Source: CAD feature listing. Evaluate the final solid. Frame: model axes, mm. A direction names the side the tool comes from. Give positions to 0.01 mm unless a question says otherwise; leave off trailing zeros. Order: outer loops, then holes, each group sorted by start corner. A loop starts at its lowest first (then second) coordinate and runs counter-clockwise, first axis right, second up. Notation, with made-up numbers: M 63.5,1 L 102.5,1 A28 cw 102.5,33 Z; hole C -8,-13 d3. An arc over 180 degrees is marked long. Answer as a JSON object with one key per item and string values. Group by question number.
1. Set-up query: faces 1 (the cylindrical face through (-2.17, -27.32, -54.76)), 2 (the flat face through (0, 0, 5)), 3 (the flat face through (4, 7, 205)). Return all of +Z, -Z, +X, -X, +Y, -Y with unobstructed straight access to the full face (end or side cutting, diameter ignored); none if empty.
2. Section query D-D (y = -28.5). Output: boundary loops of the cut face in (x, z), plus the area to 3 significant figures.
3. Section query B-B (y = 0). Output: boundary loops of the cut face in (x, z), plus the area to 3 significant figures.
4. Pin query (flat end, axial travel): P1, Ø1, axis at x = 3.5, z = 31, coming from the -Y side; P2, Ø4, axis at x = 9, z = 60, coming from the -Y side; P3, Ø8, axis at x = -3.5, z = 48.5, coming from the +Y side. Return the tip coordinate at first contact, or that it passes through.
5. Section query A-A (x = 0). Output: boundary loops of the cut face in (y, z).
6. Section query C-C (z = 127.5). Output: boundary loops of the cut face in (x, y), plus the area to 3 significant figures.
7. Material intervals for L1, parallel to Y at x = -0.75, z = 76; L2, parallel to X at y = -4, z = 145; L3, parallel to Y at x = 2.5, z = -32, sorted ascending. Write a range as [from, to].
from build123d import *

# Parameters (mm, degrees)
SKETCH_1_W          = 30
SKETCH_1_H          = 30
EXTRUDE_1_DEPTH     = 5
SKETCH_2_R          = 10
SKETCH_2_R_2        = 7.5
EXTRUDE_2_DEPTH     = 200
SKETCH_3_W          = 30
SKETCH_3_H          = 30
EXTRUDE_3_DEPTH     = 60
SKETCH_4_R          = 10
EXTRUDE_4_DEPTH     = 25
CUT_EXTRUDE_1_DEPTH = 31


with BuildPart() as part:
    # 草图1 → 凸台-拉伸1 (new body)
    with BuildSketch(Plane.XY):
        Rectangle(SKETCH_1_W, SKETCH_1_H)
    extrude(amount=EXTRUDE_1_DEPTH)

    # 草图2 → 凸台-拉伸2 (add)
    with BuildSketch(Plane.XY.offset(5)):
        Circle(SKETCH_2_R)
        Circle(SKETCH_2_R_2, mode=Mode.SUBTRACT)
    extrude(amount=EXTRUDE_2_DEPTH)

    # 草图3 → 凸台-拉伸3 (add)
    with BuildSketch(Plane(origin=(0, 0, 0), x_dir=(-1, 0, 0), z_dir=(0, 0, -1))):
        Rectangle(SKETCH_3_W, SKETCH_3_H)
    extrude(amount=EXTRUDE_3_DEPTH)

    # 草图4 → 凸台-拉伸4 (add)
    with BuildSketch(Plane.XZ.offset(15)):
        with Locations((0, -45)):
            Circle(SKETCH_4_R)
    extrude(amount=EXTRUDE_4_DEPTH)

    # 草图5 → 切除-拉伸1 (cut, through all)
    with BuildSketch(Plane.XZ.offset(15)):
        with BuildLine():
            Line((15, -45), (15, -76.870462398))
            Line((15, -76.870462398), (-15, -76.870462398))
            Line((-15, -76.870462398), (-15, -45))
            ThreePointArc((-15, -45), (0, -60), (15, -45))
        make_face()
    extrude(amount=-CUT_EXTRUDE_1_DEPTH, mode=Mode.SUBTRACT)


solid = part.part
Answer sheet:
{
 "1": {"face 1": "-Y", "face 2": "+Z", "face 3": "+Z, +X, -X, +Y, -Y"},
 "2": {"outline": "C 0,-45 d20", "area": "314 mm^2"},
 "3": {"outline": "M -15,-45 A15 ccw 15,-45 L 15,5 L 10,5 L 10,205 L 7.5,205 L 7.5,5 L -7.5,5 L -7.5,205 L -10,205 L -10,5 L -15,5 Z", "area": "2,850 mm^2"},
 "4": {"P1": "y = -9.54", "P2": "y = -7.14", "P3": "y = 10"},
 "5": {"outline": "M -40,-55 L -15,-55 L -15,-60 L 15,-60 L 15,5 L 10,5 L 10,205 L 7.5,205 L 7.5,5 L -7.5,5 L -7.5,205 L -10,205 L -10,5 L -15,5 L -15,-35 L -40,-35 Z"},
 "6": {"outline": "C 0,0 d20; hole C 0,0 d15", "area": "137 mm^2"},
 "7": {"L1": "[-9.97, -7.46], [7.46, 9.97]", "L2": "[-9.17, -6.34], [6.34, 9.17]", "L3": "[-15, 15]"}
}
